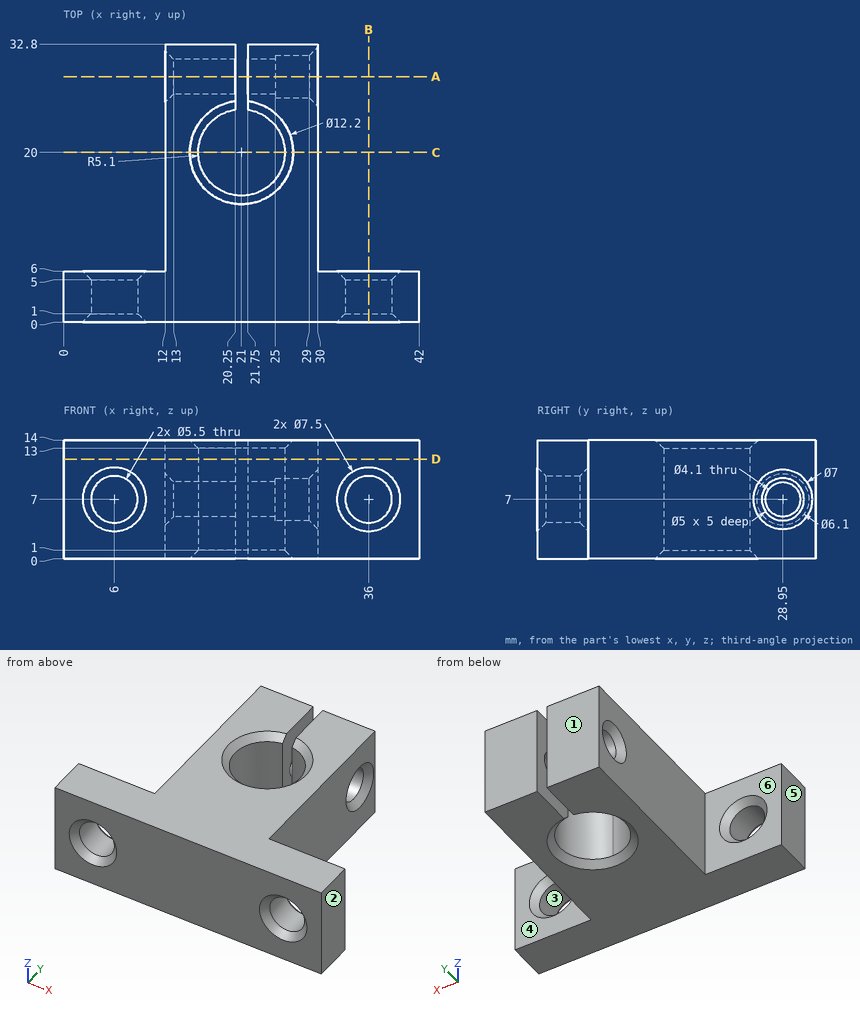
Could you check a few things on this drawing? It's one solid part, dimensions in mm from its lowest x, y, z. A direction names the side the tool comes from. Give positions to 0.01 mm unless a question says otherwise; leave off trailing zeros. Write each loop counter-clockwise with the first axis right and the second up, starting at its lowest first coordinate (ties: lowest second). Pieces come first, ordered by that corner, then holes. Notation, with made-up numbers: (-18.5, -7) -> (9.5, -7) arc R30 cw to (9.5, 25) -> close; hole circle Ø5 at (-27.5, 14.5). An arc over 180 degrees is marked (long way). Answer as CSV lines item,"result". Start each with the question number.
(1) If we section it at D-D, the plane z = 11.75: Write out the boundary of the cut face in (x, y).
(2) Please list where these lines run through material, in increasing order: line 1 (X direction, y = 3.7, z = 7); line 2 (Z direction, x = 22.6, y = 28.95); line 3 (X direction, y = 2, z = 5.5).
(3) If we mould it in two halves opening along X, with no side actions, what happens to the marked faces 1, 2 and 3? For each: +X half, -X half, draft (parallel to the pull), parting line (faces both ways), or undercut.
(4) If we section it at C-C, the plane y = 20: Write out the boundary of the cut face in (x, z), and give its area (3 significant figures).
(5) I'm going to push flat-ended pins straight in: pin 1 Ø1 at (y, z) = (7, 2) entering from -X; pin 2 Ø3.5 at (x, z) = (3, 4.5) entering from +Y; pin 3 Ø7 at (y, z) = (24, 6) entering from +X. Where does each tip first touch, or does it pass through?
(6) Which directions (+Z, -Z, +X, -X, +Y, -Y) give clear straight access to the entire face, cutting with the end or side of a thin tool? Please do the marked faces 4, 5 and 6.
(7) If we section it at A-A, the plane y = 28.95: Write out the boundary of the cut face in (x, z).
(8) If we section it at B-B, the plane x = 36: Write out the boundary of the cut face in (y, z), and give its area (3 significant figures).
Answer list:
1,outline,"(0, 0) -> (42, 0) -> (42, 6) -> (30, 6) -> (30, 32.8) -> (21.75, 32.8) -> (21.75, 25.04) arc R5.1 cw (long way) to (20.25, 25.04) -> (20.25, 32.8) -> (12, 32.8) -> (12, 6) -> (0, 6) -> close"
2,line 1,"0 to 3.25, 8.75 to 33.25, 38.75 to 42"
2,line 2,"0 to 4.95, 9.05 to 14"
2,line 3,"0 to 3.7, 8.3 to 33.7, 38.3 to 42"
3,face 1,"draft"
3,face 2,"+X half"
3,face 3,"undercut"
4,outline,"(12, 0) -> (14.9, 0) -> (15.9, 1) -> (15.9, 13) -> (14.9, 14) -> (12, 14) -> close; (26.1, 1) -> (27.1, 0) -> (30, 0) -> (30, 14) -> (27.1, 14) -> (26.1, 13) -> close"
4,area,"107 mm^2"
5,pin 1,"x = 12"
5,pin 2,"y = 6"
5,pin 3,"x = 30"
6,face 4,"+Z, -Z, +X, +Y"
6,face 5,"+Z, -Z, -X, +Y, -Y"
6,face 6,"+Z, -Z, -X, +Y"
7,outline,"(12, 0) -> (20.25, 0) -> (20.25, 4.95) -> (13, 4.95) -> (12, 3.95) -> close; (12, 10.05) -> (13, 9.05) -> (20.25, 9.05) -> (20.25, 14) -> (12, 14) -> close; (21.75, 0) -> (30, 0) -> (30, 3.5) -> (29, 4.5) -> (25, 4.5) -> (25, 4.95) -> (21.75, 4.95) -> close; (21.75, 9.05) -> (25, 9.05) -> (25, 9.5) -> (29, 9.5) -> (30, 10.5) -> (30, 14) -> (21.75, 14) -> close"
8,outline,"(0, 0) -> (6, 0) -> (6, 3.25) -> (5, 4.25) -> (1, 4.25) -> (0, 3.25) -> close; (0, 10.75) -> (1, 9.75) -> (5, 9.75) -> (6, 10.75) -> (6, 14) -> (0, 14) -> close"
8,area,"49.0 mm^2"
